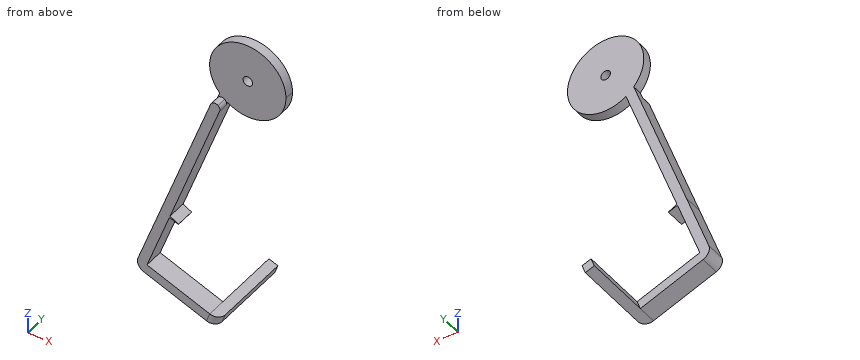
from build123d import *

# Parameters (mm, degrees)
F0_R        = 2.5
F1_DEPTH    = 5
F2_DEPTH    = 10
F3_R        = 2.49999
F4_T1_DEPTH = 35
F4_T3_DEPTH = 30
F5_SIZE2    = 0.881625
F5_SIZE     = 4.99999
F6_DEPTH    = 35


# Not quite as in the source:
# - a fillet or chamfer that OpenCascade refuses, or shapes differently, is made with other operations: its cross-section is extruded or revolved along the edge and cut away or added
# - a fillet or chamfer is up to 0.001 mm smaller than in the source, because OpenCascade refuses the exact size


with BuildPart() as f1:
    # F0 (on Front) → F1 (new body)
    with BuildSketch(Plane.XZ):
        with BuildLine():
            ThreePointArc((20, 33.8170940264), (-7.2600924867, 52.4528407806), (-14.7291057085, 20.287369527))
            ThreePointArc((-14.7291057085, 20.287369527), (-12.8011117725, 18.4505219497), (-10.6461806987, 16.8860917959))
            ThreePointArc((-10.6461806987, 16.8860917959), (9.671514515, 16.3110434442), (20, 33.8170940264))
        make_face()
        with Locations((0, 33.8170940264)):
            Circle(F0_R, mode=Mode.SUBTRACT)
        with BuildLine():
            Line((-42.3206788698, -55.5198547009), (-37.6222157658, -57.2299554175))
            Line((-37.6222157658, -57.2299554175), (-37.2801956225, -56.2902627967))
            Line((-37.2801956225, -56.2902627967), (-10.6461806987, 16.8860917959))
            ThreePointArc((-10.6461806987, 16.8860917959), (-12.8011117725, 18.4505219497), (-14.7291057085, 20.287369527))
            Line((-14.7291057085, 20.287369527), (-42.3206788698, -55.5198547009))
        make_face()
        Polygon((-37.2801956225, -56.2902627967), (-37.6222157658, -57.2299554175), (-32.9237526619, -58.9400561341), (-32.5817325186, -58.0003635134), align=None)
        Polygon((-49.362959087, -89.48738258), (-37.6222157658, -57.2299554175), (-42.3206788698, -55.5198547009), (-55.7715229075, -92.4757449673), (-51.0730598036, -94.1858456839), align=None)
        Polygon((-16.4737173595, -101.4580875964), (-49.362959087, -89.48738258), (-51.0730598036, -94.1858456839), (-18.1838180761, -106.1565507003), align=None)
        Polygon((-11.7752542555, -103.168188313), (-16.4737173595, -101.4580875964), (-18.1838180761, -106.1565507003), (-13.4853549722, -107.8666514169), align=None)
    extrude(amount=F1_DEPTH)

    # F0 (on Front) → F2 (join)
    with BuildSketch(Plane.XZ):
        with BuildLine():
            Line((-42.3206788698, -55.5198547009), (-37.6222157658, -57.2299554175))
            Line((-37.6222157658, -57.2299554175), (-37.2801956225, -56.2902627967))
            Line((-37.2801956225, -56.2902627967), (-10.6461806987, 16.8860917959))
            ThreePointArc((-10.6461806987, 16.8860917959), (-12.8011117725, 18.4505219497), (-14.7291057085, 20.287369527))
            Line((-14.7291057085, 20.287369527), (-42.3206788698, -55.5198547009))
        make_face()
        Polygon((-49.362959087, -89.48738258), (-37.6222157658, -57.2299554175), (-42.3206788698, -55.5198547009), (-55.7715229075, -92.4757449673), (-51.0730598036, -94.1858456839), align=None)
        Polygon((-16.4737173595, -101.4580875964), (-49.362959087, -89.48738258), (-51.0730598036, -94.1858456839), (-18.1838180761, -106.1565507003), align=None)
        Polygon((-11.7752542555, -103.168188313), (-16.4737173595, -101.4580875964), (-18.1838180761, -106.1565507003), (-13.4853549722, -107.8666514169), align=None)
        Polygon((-37.2801956225, -56.2902627967), (-37.6222157658, -57.2299554175), (-32.9237526619, -58.9400561341), (-32.5817325186, -58.0003635134), align=None)
    extrude(amount=F2_DEPTH)

    # F3 (radius 2.5 in the source; OpenCascade refuses exactly that, so slightly less here)
    f3_edges = [f1.edges().sort_by_distance(p)[0] for p in [
        (-10.646181, -7.5, 16.886092),
        (-14.729106, -7.5, 20.28737),
    ]]
    fillet(f3_edges, radius=F3_R)

    # F4: fillet of radius 5 on 2 edges, made by hand

    # F4_s2 → F4_t1 (cut)
    with BuildSketch(Plane.XZ.offset(-12.5)):
        with BuildLine():
            ThreePointArc((-54.0614221909, -87.7772818634), (-53.8944980222, -91.6004738887), (-51.0730598036, -94.1858456839))
            Line((-51.0730598036, -94.1858456839), (-55.7715229075, -92.4757449673))
            Line((-55.7715229075, -92.4757449673), (-54.0614221909, -87.7772818634))
        make_face()
    extrude(amount=F4_T1_DEPTH, mode=Mode.SUBTRACT)

    # F4_s4 → F4_t3 (cut)
    with BuildSketch(Plane(origin=(-40.5204121723, 0, -111.3289174704), x_dir=(0, 1, 0), z_dir=(0.3420201433, 0, 0.9396926208))):
        with BuildLine():
            ThreePointArc((-10, -19.2204790217), (-8.5355339059, -22.7560129276), (-5, -24.2204790217))
            Line((-5, -24.2204790217), (-10, -24.2204790217))
            Line((-10, -24.2204790217), (-10, -19.2204790217))
        make_face()
    extrude(amount=F4_T3_DEPTH, mode=Mode.SUBTRACT)

    # F5 (size 5 and 0.8816349035 in the source; OpenCascade refuses exactly that, so slightly less here)
    f5_edges = [f1.edges().sort_by_distance(p)[0] for p in [
        (-32.581733, -5, -58.000364),
    ]]
    chamfer(f5_edges, length=F5_SIZE, length2=F5_SIZE2)

    # F0 (on Front) → F6 (join)
    with BuildSketch(Plane.XZ):
        Polygon((-11.7752542555, -103.168188313), (-16.4737173595, -101.4580875964), (-18.1838180761, -106.1565507003), (-13.4853549722, -107.8666514169), align=None)
    extrude(amount=-F6_DEPTH)


solid = f1.part
Geometry check sheet. Reference: the model listing, model coordinates, mm. Give positions to 0.01 mm unless a question says otherwise; leave off trailing zeros. Write each loop counter-clockwise with the first axis right and the second up, starting at its lowest first coordinate (ties: lowest second). Pieces come first, ordered by that corner, then holes. Notation, with made-up numbers: (-1, 51) - (14, 51) arc R12 cw to (14, 61) - close; hole circle Ø5 at (76.5, 34.25). An arc over 180 degrees is marked (long way). Put each result on its own line as item: value.
1. Thickness scan on line 1 (Z direction, x = 0, y = -2.6); line 2 (Y direction, x = -24.5, z = -12); line 3 (X direction, y = -4, z = -33). Record the ranges inside material, lowest first.
Ans:
line 1: z = 13.82 to 31.32, 36.32 to 53.82
line 2: y = -10 to 0
line 3: x = -34.12 to -28.8
2. Sectioned sample at C-C, the plane z = -97. Enter the section's corners in (x, y).
Ans:
outline: (-43.34, -10) - (-28.72, -10) - (-28.72, 0) - (-43.34, 0) - close
3. Go/stop test with flat-tipped pins: pin 1 (4 mm diameter, centred on x = 1.5, z = 32.5, fed in from -Y); pin 2 (6 mm diameter, centred on x = -3.5, y = 3.5, fed in from -Z); pin 3 (1 mm diameter, centred on x = -44, z = -72, fed in from +Y). Record where each tip stops, or that it passes through.
Ans:
pin 1: stops at y = -5
pin 2: passes through
pin 3: stops at y = 0
4. Sectioned sample at D-D, the plane y = 16. Enter the section's corners in (x, z), plus the area to 3 significant figures.
Ans:
outline: (-18.18, -106.16) - (-13.49, -107.87) - (-11.78, -103.17) - (-16.47, -101.46) - close
area: 25.0 mm²
5. Sectioned sample at A-A, the plane x = 0. Enter the section's corners in (y, z).
Ans:
outline: (-5, 13.82) - (0, 13.82) - (0, 31.32) - (-5, 31.32) - close; (-5, 36.32) - (0, 36.32) - (0, 53.82) - (-5, 53.82) - close
